from build123d import *

# Parameters (mm, degrees)
PAD_DEPTH           = 10
SKETCH001_R         = 1.75
POCKET_DEPTH        = 15.001
SKETCH002_R         = 4
POCKET001_DEPTH     = 5
SKETCH004_W         = 15
SKETCH004_H         = 0.8
POCKET002_DEPTH     = 9
POCKET003_DEPTH     = 9
LINEARPATTERN_COUNT = 8
LINEARPATTERN_PITCH = 2


with BuildPart() as part:
    # Sketch → Pad (new body)
    with BuildSketch(Plane.XY):
        Polygon((-5, 11), (5, 11), (5, -11), (-5, -11), (-10, -2.5), (-10, 2.5), align=None)
    extrude(amount=PAD_DEPTH)

    # Sketch001 → Pocket (cut, through all)
    with BuildSketch(Plane.YZ.offset(5)):
        with Locations((-6, 5)):
            Circle(SKETCH001_R)
        with Locations((6, 5)):
            Circle(SKETCH001_R)
    extrude(amount=-POCKET_DEPTH, mode=Mode.SUBTRACT)

    # Sketch002 → Pocket001 (cut)
    with BuildSketch(Plane(origin=(-10, 0, 0), x_dir=(0, -1, 0), z_dir=(-1, 0, 0))):
        with Locations((-6, 5)):
            Circle(SKETCH002_R)
        with Locations((6, 5)):
            Circle(SKETCH002_R)
    extrude(amount=-POCKET001_DEPTH, mode=Mode.SUBTRACT)

    # Sketch004 → Pocket002 (cut)
    with BuildSketch(Plane.XY.offset(10)):
        with Locations((-2.5, 0)):
            Rectangle(SKETCH004_W, SKETCH004_H)
    extrude(amount=-POCKET002_DEPTH, mode=Mode.SUBTRACT)

    # Sketch003 → Pocket003 (cut)
    with BuildSketch(Plane.XY.offset(10)):
        with BuildLine():
            ThreePointArc((-8.9, 0.7), (-9.45, 1.25), (-10, 0.7))
            Line((-10, 0.7), (-10, 0.4))
            Line((-10, 0.4), (-8.9, 0.4))
            Line((-8.9, 0.4), (-8.9, 0.7))
        make_face()
    pocket003 = extrude(amount=-POCKET003_DEPTH, mode=Mode.SUBTRACT)

    # LinearPattern: Pocket003 ×8
    with Locations(*[(i * LINEARPATTERN_PITCH, 0, 0) for i in range(1, LINEARPATTERN_COUNT)]):
        add(pocket003, mode=Mode.SUBTRACT)


solid = part.part
Here's how the part is built. I have some questions about the finished solid (model axes, mm). A direction names the side the tool comes from. Coordinates: 2 decimals unless noted, no trailing zeros. Loops run counter-clockwise (first coordinate to the right, second up) from the corner with the lowest first, then second, coordinate; pieces in that order, holes last. Notation, with made-up numbers: (-7, 1.25) -> (21, 1.25) arc R14 cw to (21, 21.25) -> close; hole circle Ø5 at (-7.5, 65). An arc over 180 degrees is marked (long way). Use one line per item in the form item = value. Start each with the question number.
(1) Please list where these lines run through material, in increasing order: line 1 along Z through (x, y) = (0.25, -6); line 2 along Y through (x, z) = (-6.05, 5); line 3 along Z through (x, y) = (-7.7, -6).
(2) If we section it at D-D (y = 2.75): Please give me the cut outline in (x, z), then the cut area to 3 significant figures.
(3) On a 3-axis mill with a long thin cutter (end or side, diameter ignored), from which of +Z, -Z, +X, -X, +Y, -Y can I reach the whole of each face in a straight line? I mean faces 1 (the face through (3.5, 0.4, 5.6)), 2 (the face through (-5.8, -9.64, 2.71)), 3 (the face through (-1.44, 1.25, 5.56)), 4 (the face through (-7, -2, 5)). Say none if no direction works.
(4) If we section it at A-A (x = 3.5): Please give me the cut outline in (y, z), then the cut area to 3 significant figures.
(5) Will this pin go through, and if not, where does the flat tip stop? pin 1 (4 mm diameter, centred on y = 6, z = 5.5, fed in from -X).
(6) If we section it at B-B (y = 6): Please give me the cut outline in (x, z), then the cut area to 3 significant figures.
(7) We'd pull the mould along Y, two halves only. Please class faces 5 (the face through (-3.44, 1.25, 5.56)), 6 (the face through (-1, 0, 0)), 7 (the face through (0, -11, 5)): pulls with the +Y half, pulls with the -Y half, needs draft (parallel to the pull), parting line crosses it, or undercut.
(8) If we section it at C-C (x = -7.45): Please give me the cut outline in (y, z) (3 decimals).
Verdict:
q1.line_1 = 0 to 3.25, 6.75 to 10
q1.line_2 = -2 to -0.4, 0.4 to 2
q1.line_3 = 0 to 1, 9 to 10
q2.outline = (-9.85, 0) -> (5, 0) -> (5, 10) -> (-9.85, 10) -> (-9.85, 7.33) -> (-5, 7.33) -> (-5, 2.67) -> (-9.85, 2.67) -> close
q2.area = 126 mm²
q3.face_1 = +Z, +X, -X
q3.face_2 = +Z, -Z, -X, -Y
q3.face_3 = +Z
q3.face_4 = -X
q4.outline = (-11, 0) -> (11, 0) -> (11, 10) -> (0.4, 10) -> (0.4, 1) -> (-0.4, 1) -> (-0.4, 10) -> (-11, 10) -> close; hole circle Ø3.5 at (-6, 5); hole circle Ø3.5 at (6, 5)
q4.area = 194 mm²
q5.pin_1 = -5
q6.outline = (-7.94, 0) -> (5, 0) -> (5, 3.25) -> (-5, 3.25) -> (-5, 1) -> (-7.94, 1) -> close; (-7.94, 9) -> (-5, 9) -> (-5, 6.75) -> (5, 6.75) -> (5, 10) -> (-7.94, 10) -> close
q6.area = 70.9 mm²
q7.face_5 = undercut
q7.face_6 = needs draft
q7.face_7 = pulls with the -Y half
q8.outline = (-6.835, 0) -> (6.835, 0) -> (6.835, 1.088) arc R4 cw (long way) to (6.835, 8.912) -> (6.835, 10) -> (1.25, 10) -> (1.25, 1) -> (-0.4, 1) -> (-0.4, 10) -> (-6.835, 10) -> (-6.835, 8.912) arc R4 cw (long way) to (-6.835, 1.088) -> close
